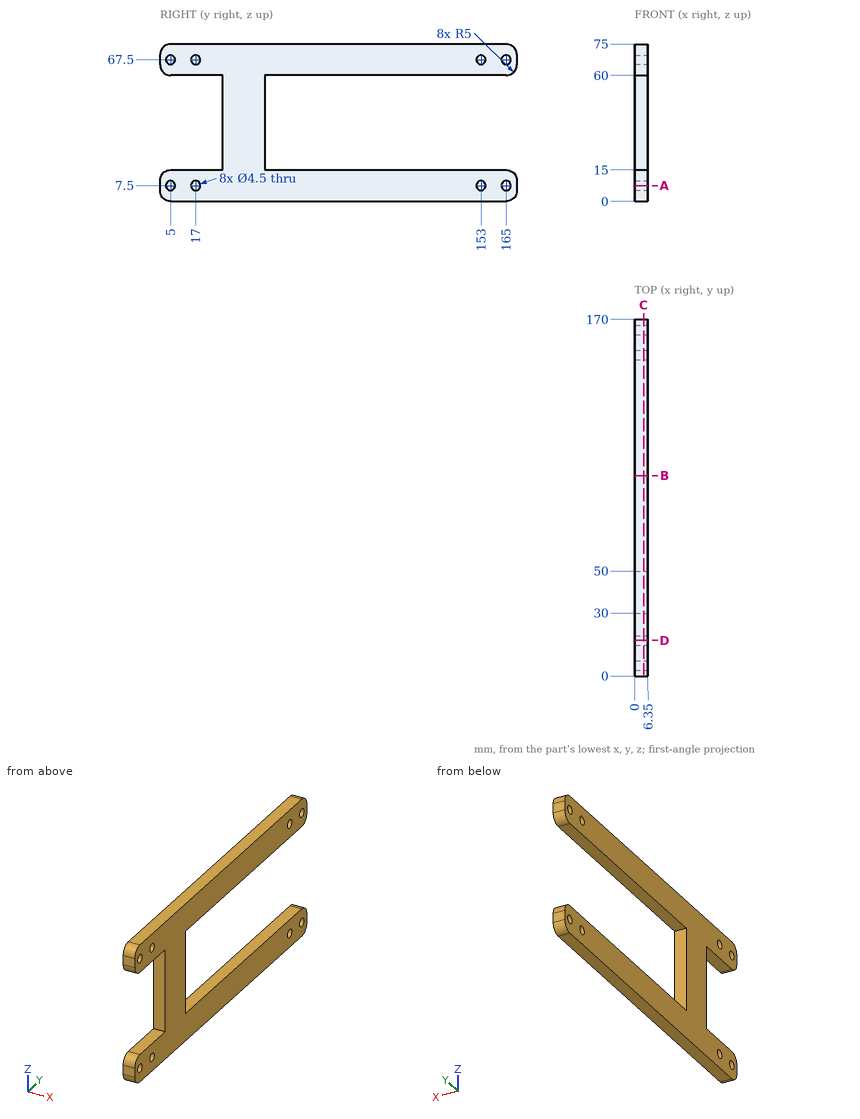
For this review, use the dimensioned drawing (mm, ordinates from the lowest corner) and the shaded views. Give positions to 0.01 mm unless a question says otherwise; leave off trailing zeros. Write each loop counter-clockwise with the first axis right and the second up, starting at its lowest first coordinate (ties: lowest second). Pieces come first, ordered by that corner, then holes.
(1) For P1, Ø3, axis at x = 2.5, z = 38.5, coming from the -Y side; P2, Ø4, axis at y = 17, z = 67.5, coming from the -X side; P3, Ø1.9, axis at x = 4, z = 29.5, coming from the +Y side, all flat-tipped, find the tip position at first contact; note any pin that passes through.
(2) Consider section D-D, the plane y = 17. Give the boundary of the cut face in (x, z), and give its area (3 significant figures).
(3) Consider section A-A, the plane z = 7.5. Give the boundary of the cut face in (x, y), and give its area (3 significant figures).
(4) Consider section B-B, the plane y = 95.5. Give the boundary of the cut face in (x, z).
(5) Consider section C-C, the plane x = 4.25. Give the number of separate pieces and of enclosed holes in the cut face, and give its area (3 significant figures).
(6) To check wall thickness, follow L1, parallel to Z at x = 3, y = 153; L2, parallel to Y at x = 3, z = 67.5; L3, parallel to Z at x = 5.5, y = 159.5. State the ranges of each line that lie inside material, in increasing order.
Returned:
1. P1: stops at y = 30
1. P2: passes through
1. P3: stops at y = 50
2. outline: (0, 0) - (6.35, 0) - (6.35, 5.25) - (0, 5.25) - close; (0, 9.75) - (6.35, 9.75) - (6.35, 15) - (0, 15) - close; (0, 60) - (6.35, 60) - (6.35, 65.25) - (0, 65.25) - close; (0, 69.75) - (6.35, 69.75) - (6.35, 75) - (0, 75) - close
2. area: 133 mm2
3. outline: (0, 0) - (6.35, 0) - (6.35, 2.75) - (0, 2.75) - close; (0, 7.25) - (6.35, 7.25) - (6.35, 14.75) - (0, 14.75) - close; (0, 19.25) - (6.35, 19.25) - (6.35, 150.75) - (0, 150.75) - close; (0, 155.25) - (6.35, 155.25) - (6.35, 162.75) - (0, 162.75) - close; (0, 167.25) - (6.35, 167.25) - (6.35, 170) - (0, 170) - close
3. area: 965 mm2
4. outline: (0, 0) - (6.35, 0) - (6.35, 15) - (0, 15) - close; (0, 60) - (6.35, 60) - (6.35, 75) - (0, 75) - close
5. separate pieces: 1
5. enclosed holes: 8
5. area: 5,830 mm2
6. L1: z = 0 to 5.25, 9.75 to 15, 60 to 65.25, 69.75 to 75
6. L2: y = 0 to 2.75, 7.25 to 14.75, 19.25 to 150.75, 155.25 to 162.75, 167.25 to 170
6. L3: z = 0 to 15, 60 to 75
